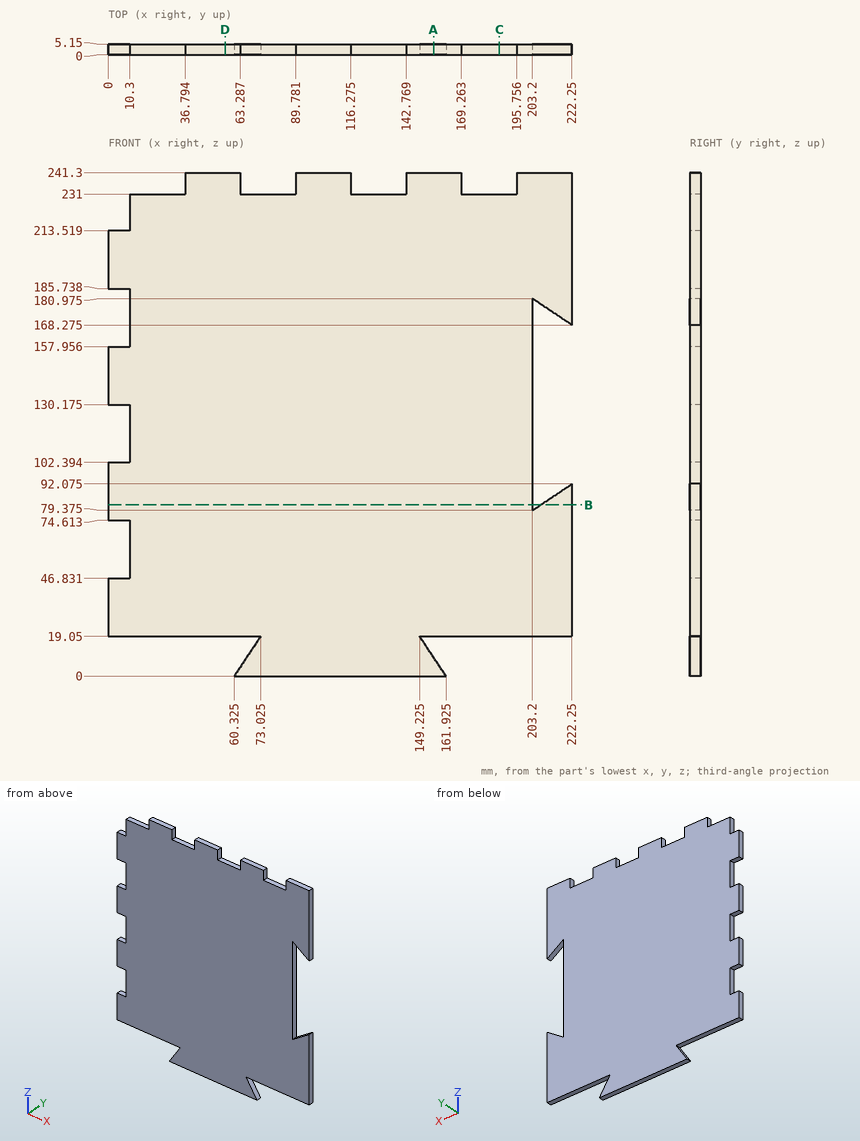
Here's the drawing with two shaded views (mm, measured from the low corner). I have some questions. Coordinates: 2 decimals unless noted, no trailing zeros. Order: outer loops, then holes, each group sorted by start corner. A loop starts at its lowest first (then second) coordinate and runs counter-clockwise, first axis right, second up.
Item 1: If we section it at C-C on x = 187.5: List the corners of the cut face in (y, z) for me.
Result sheet:
outline: (0, 19.05) - (5.15, 19.05) - (5.15, 231) - (0, 231) - close
Item 2: For P1, Ø1.5, axis at x = 17.5, y = 2, coming from the +Z side; P2, Ø2.5, axis at x = 3, y = 2, coming from the -Z side; P3, Ø2.5, axis at y = 2, z = 172, coming from the -X side, each with a flat end and sliding along its axis, tell me the tip position at first contact or that it passes through.
Result sheet:
P1: stops at z = 231
P2: stops at z = 19.05
P3: stops at x = 10.3
Item 3: If we section it at B-B on z = 82: List the corners of the cut face in (x, y) for me.
Result sheet:
outline: (0, 0) - (203.2, 0) - (203.2, 5.15) - (0, 5.15) - close; (207.14, 0) - (222.25, 0) - (222.25, 5.15) - (207.14, 5.15) - close
Item 4: If we section it at A-A on x = 156: List the corners of the cut face in (y, z) for me.
Result sheet:
outline: (0, 0) - (5.15, 0) - (5.15, 8.89) - (0, 8.89) - close; (0, 19.05) - (5.15, 19.05) - (5.15, 241.3) - (0, 241.3) - close
Item 5: I need wall thicknesses on line 1 (Z direction, x = 162.5, y = 3.55); line 2 (Z direction, x = 89, y = 4.9); line 3 (X direction, y = 2.9, z = 114). Which ranges of each line are inside material? Lowest first, please.
Result sheet:
line 1: z = 19.05 to 241.3
line 2: z = 0 to 231
line 3: x = 10.3 to 203.2
Item 6: If we section it at D-D on x = 56: List the corners of the cut face in (y, z) for me.
Result sheet:
outline: (0, 19.05) - (5.15, 19.05) - (5.15, 241.3) - (0, 241.3) - close
